from build123d import *

# Parameters (mm, degrees)
BASE_FLANGE1_DEPTH = 38.1
SKETCH2_R          = 2.5796875
CUT_EXTRUDE1_DEPTH = 219.711637617


# Sheet-metal steps are written as plain solids
with BuildPart() as part:
    # Sketch1 → Base-Flange1 (new body)
    with BuildSketch(Plane(origin=(0, 0, 0), x_dir=(1, 0, 0), z_dir=(0, 1, 0))):
        with BuildLine():
            Line((0, 0), (48.537979736, 0))
            ThreePointArc((48.537979736, 0), (50.62781396, 0.415693873), (52.399489868, 1.599489868))
            Line((52.399489868, 1.599489868), (142.807064676, 92.007064676))
            ThreePointArc((142.807064676, 92.007064676), (143.837108809, 92.695318162), (145.052128706, 92.937000646))
            Line((145.052128706, 92.937000646), (188.822000646, 92.937000646))
            ThreePointArc((188.822000646, 92.937000646), (191.067064676, 92.007064676), (191.997000646, 89.762000646))
            Line((191.997000646, 89.762000646), (191.997000646, -46.762999354))
            Line((191.997000646, -46.762999354), (194.283000646, -46.762999354))
            Line((194.283000646, -46.762999354), (194.283000646, 89.762000646))
            ThreePointArc((194.283000646, 89.762000646), (192.683510778, 93.623510778), (188.822000646, 95.223000646))
            Line((188.822000646, 95.223000646), (145.052128706, 95.223000646))
            ThreePointArc((145.052128706, 95.223000646), (142.962294482, 94.807306773), (141.190618574, 93.623510778))
            Line((141.190618574, 93.623510778), (50.783043766, 3.21593597))
            ThreePointArc((50.783043766, 3.21593597), (49.752999634, 2.527682484), (48.537979736, 2.286))
            Line((48.537979736, 2.286), (0, 2.286))
            Line((0, 2.286), (0, 0))
        make_face()
    extrude(amount=BASE_FLANGE1_DEPTH)

    # Sketch2 → Cut-Extrude1 (cut, through all)
    with BuildSketch(Plane(origin=(0, 0, -2.286), x_dir=(-1, 0, 0), z_dir=(0, 0, -1))):
        with Locations((-12.7, 19.05)):
            Circle(SKETCH2_R)
        with Locations((-38.1, 19.05)):
            Circle(SKETCH2_R)
    extrude(amount=-CUT_EXTRUDE1_DEPTH, mode=Mode.SUBTRACT)


solid = part.part
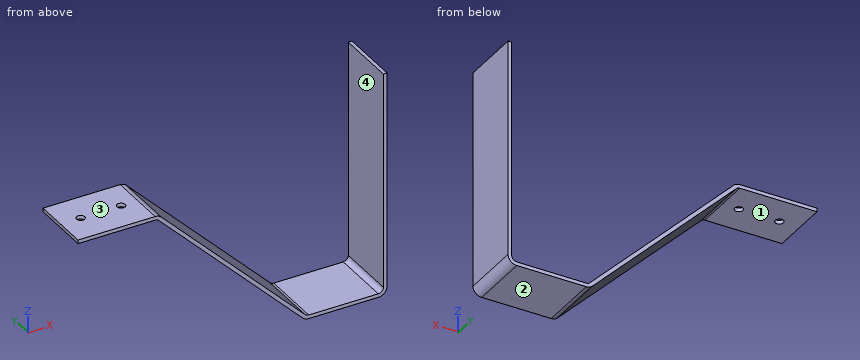
Could you check a few things on this model? Use its own coordinates, in mm. Face numbers are marked on the shaded views. A direction names the side the tool comes from. Coordinates: 2 decimals unless noted, no trailing zeros. Write each loop counter-clockwise with the first axis right and the second up, starting at its lowest first coordinate (ties: lowest second). Pieces come first, ordered by that corner, then holes. Notation, with made-up numbers: (67, 6) - (77, 6) arc R13 cw to (77, 20) - close; hole circle Ø5 at (-15.5, -39). An arc over 180 degrees is marked (long way). Put each result on its own line as item: value. Start each with the question number.
Q1. Which directions (+Z, -Z, +X, -X, +Y, -Y) give clear straight access to the entire face, cutting with the end or side of a thin tool? Please do the marked faces 1, 2, 3 and 4.
Q2. I want a section at D-D on x = 154.5. Write out the boundary of the cut face in (y, z).
Q3. I want a section at B-B on y = 19.05. Write out the boundary of the cut face in (x, z) (3 decimals).
Q4. I'm going to push flat-ended pins straight in: P1, Ø11.5, axis at x = 162, y = 26.5, coming from the +Z side; P2, Ø5, axis at x = 27, y = 18.5, coming from the -Z side; P3, Ø2, axis at x = 96.5, y = 18, coming from the -Z side. Where does each tip first touch, or does it pass through?
Q5. Please list where these lines run through material, in increasing order: L1, parallel to Y at x = 38.1, z = -0.6; L2, parallel to X at y = 19, z = -1; L3, parallel to X at y = 3, z = 10.
Q6. I want a section at C-C on z = -77. Write out the boundary of the cut face in (x, y).
Q7. I want a section at A-A on x = 38.1. Write out the boundary of the cut face in (y, z), plus the area to 3 significant figures.
Checks:
1. face 1: -Z, -X, +Y, -Y
1. face 2: -Z, +X, -X, +Y, -Y
1. face 3: +Z, -X, +Y, -Y
1. face 4: +Z, +Y, -Y
2. outline: (0, -95.22) - (38.1, -95.22) - (38.1, -92.94) - (0, -92.94) - close
3. outline: (0, -2.286) - (10.12, -2.286) - (10.12, 0) - (0, 0) - close; (15.28, -2.286) - (35.52, -2.286) - (35.52, 0) - (15.28, 0) - close; (40.68, -2.286) - (48.538, -2.286) arc R3.175 cw to (50.783, -3.216) - (141.191, -93.624) arc R5.461 ccw to (145.052, -95.223) - (188.822, -95.223) arc R5.461 ccw to (194.283, -89.762) - (194.283, 46.763) - (191.997, 46.763) - (191.997, -89.762) arc R3.175 cw to (188.822, -92.937) - (145.052, -92.937) arc R3.175 cw to (142.807, -92.007) - (52.399, -1.599) arc R5.461 ccw to (48.538, 0) - (40.68, 0) - close
4. P1: z = -92.94
4. P2: z = -2.29
4. P3: z = -49.93
5. L1: 0 to 16.47, 21.63 to 38.1
5. L2: 0 to 10.12, 15.28 to 35.52, 40.68 to 51.69, 192 to 194.28
5. L3: 192 to 194.28
6. outline: (124.57, 0) - (127.8, 0) - (127.8, 38.1) - (124.57, 38.1) - close; (192, 0) - (194.28, 0) - (194.28, 38.1) - (192, 38.1) - close
7. outline: (0, -2.29) - (16.47, -2.29) - (16.47, 0) - (0, 0) - close; (21.63, -2.29) - (38.1, -2.29) - (38.1, 0) - (21.63, 0) - close
7. area: 75.3 mm²
